```python
from build123d import *

# Parameters (mm, degrees)
F0_W     = 100
F0_H     = 200
F1_DEPTH = 5
F2_W     = 50
F2_H     = 40
F3_DEPTH = 25
F5_D     = 25


with BuildPart() as f1:
    # F0 (on Top) → F1 (new body)
    with BuildSketch(Plane.XY):
        Rectangle(F0_W, F0_H)
    extrude(amount=F1_DEPTH)

    # F2 (on face) → F3 (join)
    with BuildSketch(Plane.XY.offset(5)):
        with Locations((-25, -80)):
            Rectangle(F2_W, F2_H)
    extrude(amount=F3_DEPTH)

    # F5 (through all)
    with Locations(Plane.XY.offset(5)):
        with Locations((-15, 70)):
            Hole(F5_D / 2)


solid = f1.part
```
Geometry check sheet. Reference: the model listing, model coordinates, mm. A direction names the side the tool comes from. Coordinates: 2 decimals unless noted, no trailing zeros. Loops run counter-clockwise (first coordinate to the right, second up) from the corner with the lowest first, then second, coordinate; pieces in that order, holes last.
Item 1: Sectioned sample at C-C, the plane x = -15. Record the boundary of the cut face in (y, z), then the cut area to 4 significant figures.
Item 2: Sectioned sample at D-D, the plane y = -87. Record the boundary of the cut face in (x, z).
Item 3: Thickness scan on line 1 (Y direction, x = -15, z = 1.6); line 2 (Z direction, x = 13, y = 87); line 3 (Y direction, x = -31.5, z = 7.5). Record the ranges inside material, lowest first.
Item 4: Sectioned sample at B-B, the plane y = 70. Record the boundary of the cut face in (x, z).
Item 5: Access from +Z, -Z, +X, -X, +Y, -Y to the whole of each face (thin tool, end or side, straight path). Record for faces 1 (the face through (-25, -60, 17)), 2 (the face through (0, -80, 17)), 3 (the face through (-12, -100, 11)).
Item 6: Sectioned sample at A-A, the plane x = -5. Record the boundary of the cut face in (y, z), then the cut area to 4 significant figures.
Item 7: Go/stop test with flat-tipped pins: pin 1 Ø3 at (x, y) = (-6, 26.5) entering from +Z; pin 2 Ø2 at (y, z) = (-80, 6.5) entering from +X. Record where each tip stops, or that it passes through.
Check result:
1. outline: (-100, 0) - (57.5, 0) - (57.5, 5) - (-60, 5) - (-60, 30) - (-100, 30) - close; (82.5, 0) - (100, 0) - (100, 5) - (82.5, 5) - close
1. area: 1,875 mm2
2. outline: (-50, 0) - (50, 0) - (50, 5) - (0, 5) - (0, 30) - (-50, 30) - close
3. line 1: y = -100 to 57.5, 82.5 to 100
3. line 2: z = 0 to 5
3. line 3: y = -100 to -60
4. outline: (-50, 0) - (-27.5, 0) - (-27.5, 5) - (-50, 5) - close; (-2.5, 0) - (50, 0) - (50, 5) - (-2.5, 5) - close
5. face 1: +Z, +X, -X, +Y
5. face 2: +Z, +X, +Y, -Y
5. face 3: +Z, -Z, +X, -X, -Y
6. outline: (-100, 0) - (62.5, 0) - (62.5, 5) - (-60, 5) - (-60, 30) - (-100, 30) - close; (77.5, 0) - (100, 0) - (100, 5) - (77.5, 5) - close
6. area: 1,925 mm2
7. pin 1: stops at z = 5
7. pin 2: stops at x = 0
